```python
from build123d import *

# Parameters (mm, degrees)
SKETCH1_W           = 10.04
SKETCH1_H           = 8.04
BOSS_EXTRUDE1_DEPTH = 3
BOSS_EXTRUDE2_START = 3
BOSS_EXTRUDE2_DEPTH = 3
FILLET2_R           = 1


with BuildPart() as part:
    # Sketch1 → Boss-Extrude1 (new body)
    with BuildSketch(Plane(origin=(0, 0, 0), x_dir=(1, 0, 0), z_dir=(0, 1, 0))):
        Rectangle(SKETCH1_W, SKETCH1_H)
    extrude(amount=BOSS_EXTRUDE1_DEPTH)

    # Sketch1<3> → Boss-Extrude2 (add)
    with BuildSketch(Plane(origin=(0, 0, 0), x_dir=(1, 0, 0), z_dir=(0, 1, 0)).offset(BOSS_EXTRUDE2_START)):
        Polygon((-2, 0.02), (-2, 4.02), (2, 4.02), (2, 0.02), (3.52, 0.02), (3.52, -1.98), (-3.52, -1.98), (-3.52, 0.02), align=None)
        Polygon((-2, 0.02), (-2, 1.54), (-3.52, 0.02), align=None)
        Polygon((3.52, 0.02), (2, 1.54), (2, 0.02), align=None)
    extrude(amount=BOSS_EXTRUDE2_DEPTH)

    # Fillet2
    fillet2_edges = [part.edges().sort_by_distance(p)[0] for p in [
        (5.02, 1.5, -4.02),
        (-5.02, 1.5, -4.02),
        (-5.02, 1.5, 4.02),
        (5.02, 1.5, 4.02),
    ]]
    fillet(fillet2_edges, radius=FILLET2_R)


solid = part.part
```
Check sheet for the modelled part. Datum: model origin and axes. Units: mm. A direction names the side the tool comes from. Give positions to 0.01 mm unless a question says otherwise; leave off trailing zeros. Loops run counter-clockwise (first coordinate to the right, second up) from the corner with the lowest first, then second, coordinate; pieces in that order, holes last. Notation, with made-up numbers: M 31.25,-1 L 50.25,-1 A29 ccw 50.25,30 Z; hole C 65,19 d2. An arc over 180 degrees is marked long. Answer in a Markdown table with one row per item.
1) Thickness scan on line 1 (X direction, y = 3.45, z = 1.75); line 2 (Z direction, x = 0.25, y = 4.2); line 3 (Y direction, x = 3, z = -2). Record the ranges inside material, lowest first.
Solutions:
| item | result |
|---|---|
| line 1 | x = -3.52 to 3.52 |
| line 2 | z = -4.02 to 1.98 |
| line 3 | y = 0 to 3 |
2) Cross-section at C-C (z = 3.5). Enter the section's corners in (x, y), plus the area to 3 significant figures.
Solutions:
| item | result |
|---|---|
| outline | M -4.9,0 L 4.9,0 L 4.9,3 L -4.9,3 Z |
| area | 29.4 mm^2 |
3) Depth check by flat-ended pin: pin 1 (1.6 mm diameter, centred on y = 5, z = 1, fed in from -X); pin 2 (2 mm diameter, centred on y = 4.5, z = -2, fed in from +X); pin 3 (1.2 mm diameter, centred on y = 5, z = -2.5, fed in from -X). Enter the tip coordinate at first touch or a pass-through.
Solutions:
| item | result |
|---|---|
| pin 1 | stops at x = -3.52 |
| pin 2 | stops at x = 2.54 |
| pin 3 | stops at x = -2 |
4) Cross-section at A-A (y = 5.3). Enter the section's corners in (x, z).
Solutions:
| item | result |
|---|---|
| outline | M -3.52,-0.02 L -2,-1.54 L -2,-4.02 L 2,-4.02 L 2,-1.54 L 3.52,-0.02 L 3.52,1.98 L -3.52,1.98 Z |
5) Cross-section at B-B (x = 2.5). Enter the section's corners in (y, z), plus the area to 3 significant figures.
Solutions:
| item | result |
|---|---|
| outline | M 0,-4.02 L 3,-4.02 L 3,-1.04 L 6,-1.04 L 6,1.98 L 3,1.98 L 3,4.02 L 0,4.02 Z |
| area | 33.2 mm^2 |
6) Cross-section at D-D (x = 1). Enter the section's corners in (y, z), plus the area to 3 significant figures.
Solutions:
| item | result |
|---|---|
| outline | M 0,-4.02 L 6,-4.02 L 6,1.98 L 3,1.98 L 3,4.02 L 0,4.02 Z |
| area | 42.1 mm^2 |
7) Tool access check on faces 1 (the face through (-2, 4, -3)), 2 (the face through (3.52, 4, 1)), 3 (the face through (0, 4, 1.98)), 4 (the face through (2, 4, -3)). Record the directions out of +Z, -Z, +X, -X, +Y, -Y that give a thin tool (end or side, any length) a straight path to the whole face; none if there is none.
Solutions:
| item | result |
|---|---|
| face 1 | -Z, -X, +Y |
| face 2 | +Z, -Z, +X, +Y |
| face 3 | +Z, +X, -X, +Y |
| face 4 | -Z, +X, +Y |
